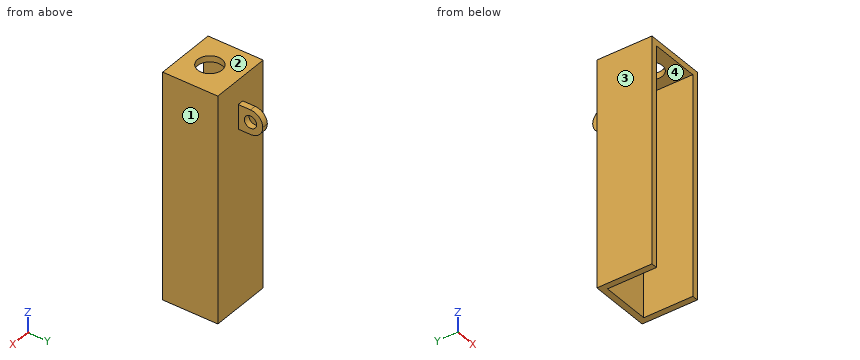
from build123d import *

# Parameters (mm, degrees)
SKETCH1_W           = 31.75
SKETCH1_H           = 28.575
BOSS_EXTRUDE1_DEPTH = 3.175
SKETCH2_R           = 6.35
CUT_EXTRUDE1_DEPTH  = 28.423991451
BOSS_EXTRUDE2_DEPTH = 114.3
SKETCH4_W           = 3.175
SKETCH4_H           = 12.7
BOSS_EXTRUDE3_DEPTH = 12.7
SKETCH5_R           = 3.175
CUT_EXTRUDE2_DEPTH  = 119.165117032


with BuildPart() as part:
    # Sketch1 → Boss-Extrude1 (new body)
    with BuildSketch(Plane.XY):
        with Locations((-5.47882926, -2.624290504)):
            Rectangle(SKETCH1_W, SKETCH1_H)
    extrude(amount=BOSS_EXTRUDE1_DEPTH)

    # Sketch2 → Cut-Extrude1 (cut, through all)
    with BuildSketch(Plane.XY.offset(3.175)):
        with Locations((-5.47882926, -4.211790504)):
            Circle(SKETCH2_R)
    extrude(amount=-CUT_EXTRUDE1_DEPTH, mode=Mode.SUBTRACT)

    # Sketch3 → Boss-Extrude2 (add)
    with BuildSketch(Plane(origin=(0, 0, 0), x_dir=(-1, 0, 0), z_dir=(0, 0, -1))):
        Polygon((21.35382926, -16.911790504), (18.17882926, -16.911790504), (18.17882926, 8.488209496), (-7.22117074, 8.488209496), (-7.22117074, -16.911790504), (-10.39617074, -16.911790504), (-10.39617074, 11.663209496), (21.35382926, 11.663209496), align=None)
    extrude(amount=BOSS_EXTRUDE2_DEPTH)

    # Sketch4 → Boss-Extrude3 (add)
    with BuildSketch(Plane(origin=(0, 11.663209496, 0), x_dir=(1, 0, 0), z_dir=(0, 1, 0))):
        with Locations((-5.47882926, 15.875)):
            Rectangle(SKETCH4_W, SKETCH4_H)
    extrude(amount=BOSS_EXTRUDE3_DEPTH)

    # Sketch5 → Cut-Extrude2 (cut, through all)
    with BuildSketch(Plane(origin=(-3.89132926, 0, 0), x_dir=(0, 0, -1), z_dir=(1, 0, 0))):
        with BuildLine():
            ThreePointArc((15.875, 24.363209496), (20.365128061, 22.503337556), (22.225, 18.013209496))
            Line((22.225, 18.013209496), (22.225, 24.363209496))
            Line((22.225, 24.363209496), (15.875, 24.363209496))
        make_face()
        with BuildLine():
            ThreePointArc((9.525, 18.013209496), (11.384871939, 22.503337556), (15.875, 24.363209496))
            Line((15.875, 24.363209496), (9.525, 24.363209496))
            Line((9.525, 24.363209496), (9.525, 18.013209496))
        make_face()
        with Locations(Location((15.875, 18.013209496, 0), (0, 0, 90))):
            Circle(SKETCH5_R)
    extrude(amount=-CUT_EXTRUDE2_DEPTH, mode=Mode.SUBTRACT)


solid = part.part
Here's how the part is built. I have some questions about the finished solid (model axes, mm). Face numbers are marked on the shaded views. Round coordinates to 2 decimals unless told otherwise and drop trailing zeros. Loops run counter-clockwise (first coordinate to the right, second up) from the corner with the lowest first, then second, coordinate; pieces in that order, holes last. Notation, with made-up numbers: (-16, 31) - (-2, 31) arc R19 cw to (-2, 39) - close; hole circle Ø7 at (-12.5, 71). An arc over 180 degrees is marked (long way). One line per question, with ' | ' between items. Start each with the question number.
Q1. I want a section at D-D (z = -14). Write out the boundary of the cut face in (x, y), then the cut area to 3 significant figures.
Q2. Please list where these lines run through material, in increasing order: line 1 (X direction, y = 1, z = -29); line 2 (Y direction, x = -13, z = -74); line 3 (Z direction, x = -13.5, y = 3) (3 decimals). Write a range as [from, to].
Q3. I want a section at A-A (x = -6). Write out the boundary of the cut face in (y, z) (3 decimals).
Q4. We'd pull the mould along X, two halves only. Please class the marked faces 1, 2, 3 and 4: +X half, -X half, draft (parallel to the pull), parting line (faces both ways), or undercut.
Q5. I want a section at B-B (z = -88). Write out the boundary of the cut face in (x, y).
Q6. I want a section at C-C (y = -1). Write out the boundary of the cut face in (x, z) (3 decimals).
Q7. Will these pins go through, and if not, where does the flat tip stop? pin 1 (4 mm diameter, centred on y = 16, z = -17, fed in from -X); pin 2 (3.5 mm diameter, centred on x = -5, y = 15.5, fed in from +Z) (3 decimals); pin 3 (4 mm diameter, centred on x = -1, y = -5.5, fed in from -Z); pin 4 (8 mm diameter, centred on y = 17.5, z = -27, fed in from +X).
Response values:
1) outline: (-21.35, -16.91) - (-18.18, -16.91) - (-18.18, 8.49) - (7.22, 8.49) - (7.22, -16.91) - (10.4, -16.91) - (10.4, 11.66) - (-3.89, 11.66) - (-3.89, 15.45) - (-7.07, 15.45) - (-7.07, 11.66) - (-21.35, 11.66) - close; (-7.07, 20.58) - (-3.89, 20.58) - (-3.89, 24.08) - (-7.07, 24.08) - close | area: 285 mm²
2) line 1: x = [-21.35, -18.18], [7.22, 10.4] | line 2: y = [8.49, 11.66] | line 3: z = [0, 3.175]
3) outline: (-16.912, 0) - (-10.54, 0) - (-10.54, 3.175) - (-16.912, 3.175) - close; (2.117, 0) - (8.488, 0) - (8.488, -114.3) - (11.663, -114.3) - (11.663, -22.225) - (18.013, -22.225) arc R6.35 ccw to (18.013, -9.525) - (11.663, -9.525) - (11.663, 3.175) - (2.117, 3.175) - close; hole circle Ø6.35 at (18.013, -15.875)
4) face 1: +X half | face 2: draft | face 3: -X half | face 4: undercut
5) outline: (-21.35, -16.91) - (-18.18, -16.91) - (-18.18, 8.49) - (7.22, 8.49) - (7.22, -16.91) - (10.4, -16.91) - (10.4, 11.66) - (-21.35, 11.66) - close
6) outline: (-21.354, -114.3) - (-18.179, -114.3) - (-18.179, 0) - (-10.957, 0) - (-10.957, 3.175) - (-21.354, 3.175) - close; (-0.001, 0) - (7.221, 0) - (7.221, -114.3) - (10.396, -114.3) - (10.396, 3.175) - (-0.001, 3.175) - close
7) pin 1: stops at x = -7.07 | pin 2: stops at z = -9.525 | pin 3: stops at z = 0 | pin 4: passes through
